```python
from build123d import *

# Parameters (mm, degrees)
SKETCH1_R               = 125
BOSS_EXTRUDE1_DEPTH     = 400
SKETCH2_W               = 100
SKETCH2_H               = 250
CUT_EXTRUDE1_DEPTH      = 200
SKETCH4_R               = 50
CUT_EXTRUDE3_DEPTH      = 60
SKETCH7_R               = 25
CUT_EXTRUDE6_DEPTH      = 176
CUT_EXTRUDE6_DEPTH_BACK = 76
FILLET2_R               = 10
SKETCH8_R               = 45
SKETCH8_R_2             = 25
CUT_EXTRUDE7_DEPTH      = 10
SKETCH10_R              = 45
SKETCH10_R_2            = 25
CUT_EXTRUDE8_DEPTH      = 10


with BuildPart() as part:
    # Sketch1 → Boss-Extrude1 (new body)
    with BuildSketch(Plane(origin=(0, 0, 0), x_dir=(1, 0, 0), z_dir=(0, 1, 0))):
        Circle(SKETCH1_R)
    extrude(amount=BOSS_EXTRUDE1_DEPTH)

    # Sketch2 → Cut-Extrude1 (cut)
    with BuildSketch(Plane(origin=(0, 400, 0), x_dir=(1, 0, 0), z_dir=(0, 1, 0))):
        Rectangle(SKETCH2_W, SKETCH2_H)
    extrude(amount=-CUT_EXTRUDE1_DEPTH, mode=Mode.SUBTRACT)

    # Sketch4 → Cut-Extrude3 (cut)
    with BuildSketch(Plane.XZ):
        Circle(SKETCH4_R)
    extrude(amount=-CUT_EXTRUDE3_DEPTH, mode=Mode.SUBTRACT)

    # Sketch7 → Cut-Extrude6 (cut, two sides)
    with BuildSketch(Plane(origin=(-50, 0, 0), x_dir=(0, 0, -1), z_dir=(1, 0, 0))) as cut_extrude6_sk:
        with BuildLine():
            Line((-87.177978871, 400), (-114.564392374, 400))
            Line((-114.564392374, 400), (-114.564392374, 335))
            ThreePointArc((-114.564392374, 335), (-105.977573518, 369.651471545), (-87.177978871, 400))
        make_face()
        with BuildLine():
            ThreePointArc((87.177978871, 400), (105.977573518, 369.651471545), (114.564392374, 335))
            Line((114.564392374, 335), (114.564392374, 400))
            Line((114.564392374, 400), (87.177978871, 400))
        make_face()
        with Locations((0, 325)):
            Circle(SKETCH7_R)
    extrude(amount=CUT_EXTRUDE6_DEPTH, mode=Mode.SUBTRACT)
    extrude(cut_extrude6_sk.sketch, amount=-CUT_EXTRUDE6_DEPTH_BACK, mode=Mode.SUBTRACT)

    # Fillet2
    fillet2_edges = [part.edges().sort_by_distance(p)[0] for p in [
        (115.807589436, 400, 47.048934409),
        (-125, 400, 0),
    ]]
    fillet(fillet2_edges, radius=FILLET2_R)

    # Sketch8 → Cut-Extrude7 (cut)
    with BuildSketch(Plane(origin=(-125, 0, 0), x_dir=(0, 0, -1), z_dir=(1, 0, 0))):
        with Locations((0, 325)):
            Circle(SKETCH8_R)
        with Locations((0, 325)):
            Circle(SKETCH8_R_2, mode=Mode.SUBTRACT)
    extrude(amount=CUT_EXTRUDE7_DEPTH, mode=Mode.SUBTRACT)

    # Sketch10 → Cut-Extrude8 (cut)
    with BuildSketch(Plane.ZY.offset(-125)):
        with Locations((0, 325)):
            Circle(SKETCH10_R)
        with Locations((0, 325)):
            Circle(SKETCH10_R_2, mode=Mode.SUBTRACT)
    extrude(amount=CUT_EXTRUDE8_DEPTH, mode=Mode.SUBTRACT)


solid = part.part
```
Source: CAD feature listing. Evaluate the final solid. Frame: model axes, mm. A direction names the side the tool comes from. Give positions to 0.01 mm unless a question says otherwise; leave off trailing zeros. Order: outer loops, then holes, each group sorted by start corner. A loop starts at its lowest first (then second) coordinate and runs counter-clockwise, first axis right, second up.
(1) Material intervals for line 1 along Y through (x, z) = (-85, 0); line 2 along X through (y, z) = (369.5, -69); line 3 along X through (y, z) = (202.5, 73), sorted ascending.
(2) Pull-direction query (X, two-part tool) for faces 1 (the face through (-82.045, 349.787, 3.255)), 2 (the face through (115, 306, 19)), 3 (the face through (50, 279, 2)), 4 (the face through (-50, 279, 2)); classes: +X half, -X half, draft (parallel to the pull), parting line (faces both ways), or undercut.
(3) Access query for faces 5 (the face through (-1, 200, -2)), 6 (the face through (-116.74, 338.52, -42.92)), 7 (the face through (116.74, 338.52, 42.92)), 8 (the face through (119.228, 192.27, -37.547)), 9 (the face through (-1, 60, 1)). Directions: +Z, -Z, +X, -X, +Y, -Y. A direction counts if a zero-diameter tool reaches every point of the face in a straight line with its end or side. Return the directions, or none.
(4) Section query A-A (z = 0). State how many separate pieces and enclosed holes the cut face has, plus the area to 3 significant figures.
(5) Section query B-B (x = 0). Return the cut outline in (y, z), plus the area to 3 significant figures.
(6) Contact query for flat-ended pins moving along their axis: P1, Ø1.5, axis at y = 309.5, z = 71.5, coming from the +X side; P2, Ø5, axis at x = 76, y = 258.5, coming from the -Z side; P3, Ø10, axis at y = 71, z = -80, coming from the +X side. Output: stop coordinate, or through.
(7) Section query D-D (y = 268.5). Return the cut outline in (x, z), plus the area to 3 significant figures.
(8) Section query C-C (y = 325). Return the cut outline in (x, z).
Outcome:
1. line 1: y = 0 to 300, 350 to 400
1. line 2: x = -104.23 to -50, 50 to 104.23
1. line 3: x = -101.47 to -50, 50 to 101.47
2. face 1: draft
2. face 2: +X half
2. face 3: undercut
2. face 4: undercut
3. face 5: +Z, -Z, +Y
3. face 6: -X
3. face 7: +X
3. face 8: +Y, -Y
3. face 9: -Y
4. separate pieces: 3
4. enclosed holes: 0
4. area: 65,700 mm2
5. outline: (0, -125) - (200, -125) - (200, 125) - (0, 125) - (0, 50) - (60, 50) - (60, -50) - (0, -50) - close
5. area: 44,000 mm2
6. P1: stops at x = 103.05
6. P2: stops at z = -101.11
6. P3: stops at x = 100
7. outline: (-50, -114.56) - (-50, 114.56) arc R125 ccw to start; (50, -114.56) arc R125 ccw to (50, 114.56) - close
7. area: 24,800 mm2
8. outline: (-116.62, -45) arc R125 ccw to (-50, -114.56) - (-50, -25) - (-115, -25) - (-115, -45) - close; (-116.62, 45) - (-115, 45) - (-115, 25) - (-50, 25) - (-50, 114.56) arc R125 ccw to start; (50, -114.56) arc R125 ccw to (116.62, -45) - (115, -45) - (115, -25) - (50, -25) - close; (50, 25) - (115, 25) - (115, 45) - (116.62, 45) arc R125 ccw to (50, 114.56) - close
